The drawing under review shows one solid part. Ordinate dimensions are in mm from its lowest x, y, z. A direction names the side the tool comes from. Give positions to 0.01 mm unless a question says otherwise; leave off trailing zeros. Write each loop counter-clockwise with the first axis right and the second up, starting at its lowest first coordinate (ties: lowest second). Pieces come first, ordered by that corner, then holes. Notation, with made-up numbers: (35, 66.25) -> (43, 66.25) arc R18 cw to (43, 101.25) -> close; hole circle Ø1 at (82.5, -13.75). An arc over 180 degrees is marked (long way). Use CSV: the item, a comma, the result in double quotes.
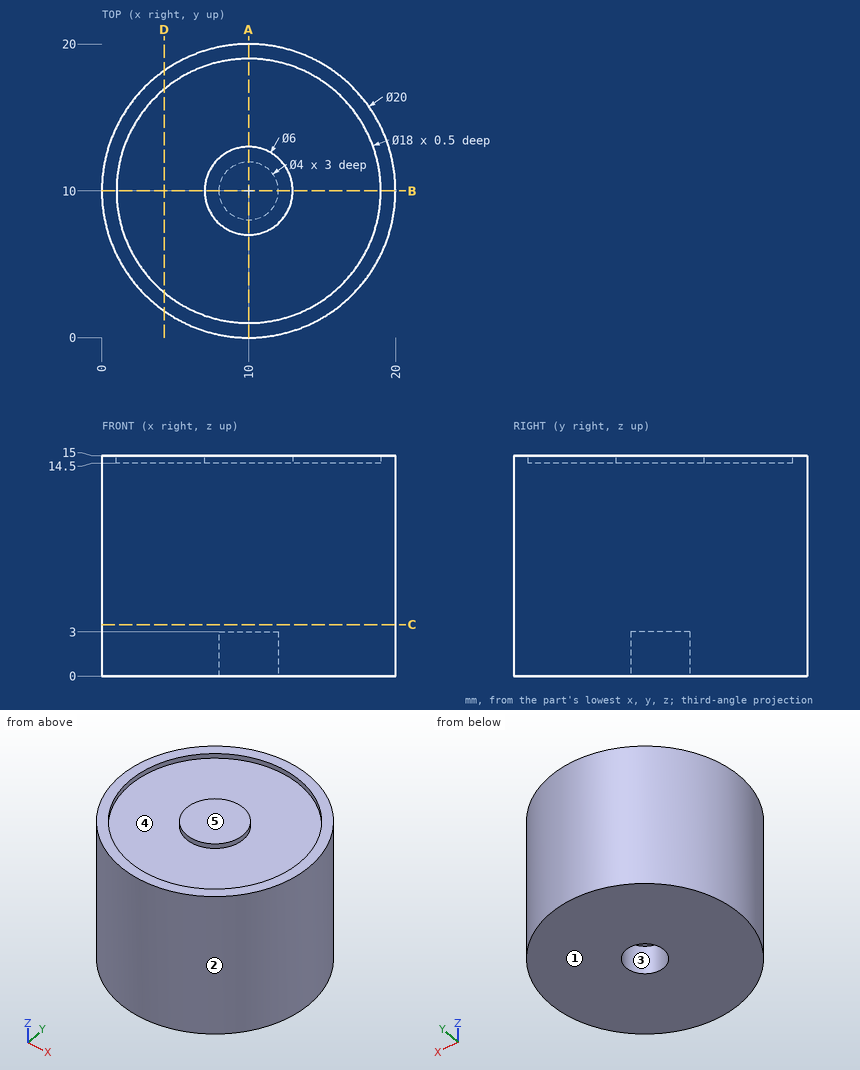
(1) Take a section at A-A (x = 10). Write out the cut boundary in (y, z).
Established:
outline,"(0, 0) -> (8, 0) -> (8, 3) -> (12, 3) -> (12, 0) -> (20, 0) -> (20, 15) -> (19, 15) -> (19, 14.5) -> (13, 14.5) -> (13, 15) -> (7, 15) -> (7, 14.5) -> (1, 14.5) -> (1, 15) -> (0, 15) -> close"
(2) Take a section at C-C (z = 3.5). Write out the cut boundary in (x, y), then the cut area to 3 significant figures.
Established:
outline,"circle Ø20 at (10, 10)"
area,"314 mm2"
(3) Take a section at D-D (x = 4.25). Write out the cut boundary in (y, z), then the cut area to 3 significant figures.
Established:
outline,"(1.82, 0) -> (18.18, 0) -> (18.18, 15) -> (16.92, 15) -> (16.92, 14.5) -> (3.08, 14.5) -> (3.08, 15) -> (1.82, 15) -> close"
area,"239 mm2"
(4) Mouldability with a two-part tool opening along Y and no side actions: class the marked faces 1, 2 and 3 as +Y half, -Y half, draft (parallel to the pull), parting line (faces both ways), or undercut.
Established:
face 1,"draft"
face 2,"parting line"
face 3,"undercut"
(5) Tool access review of the marked faces 4 and 5: name each direction out of +Z, -Z, +X, -X, +Y, -Y from which nothing blocks a thin tool from reaching the whole face with its end or side.
Established:
face 4,"+Z"
face 5,"+Z, +X, -X, +Y, -Y"
(6) For line 1 along Y through (x, z) = (10, 14.8); line 2 along Y through (x, z) = (10, 2); line 3 along Z through (x, y) = (6.75, 5.5), list the stretches that pass through material, from the lowest coordinate up. Write a range as [from, to].
Established:
line 1,"y = [0, 1], [7, 13], [19, 20]"
line 2,"y = [0, 8], [12, 20]"
line 3,"z = [0, 14.5]"
(7) Clearance check with flat-ended pins moving along their axes: pin 1 (4 mm diameter, centred on x = 6, z = 10.5, fed in from +Y); pin 2 (1 mm diameter, centred on x = 16.5, z = 7.5, fed in from +Y); pin 3 (3.5 mm diameter, centred on x = 10, y = 10, fed in from -Z). State where each tip first meets the part, or that it passes through.
Established:
pin 1,"stops at y = 19.8"
pin 2,"stops at y = 18"
pin 3,"stops at z = 3"
